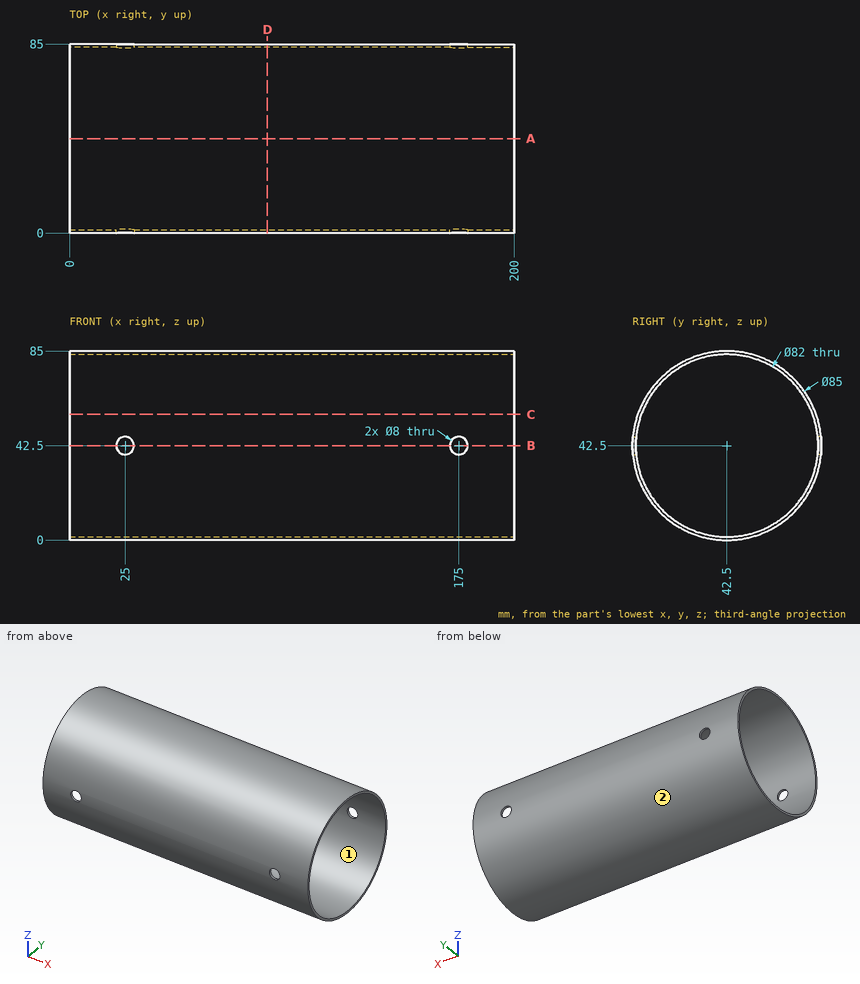
Could you check a few things on this drawing? It's one solid part, dimensions in mm from its lowest x, y, z. Coordinates: 2 decimals unless noted, no trailing zeros. Order: outer loops, then holes, each group sorted by start corner. A loop starts at its lowest first (then second) coordinate and runs counter-clockwise, first axis right, second up. Notation, with made-up numbers: M -34.5,45 L -26.5,45 A11 ccw -26.5,61 Z; hole C 72.5,42 d5. An arc over 180 degrees is marked long. Answer as a JSON object with one key per item and string values. Group by question number.
(1) Suppose I cut it at A-A, the plane y = 42.5. Please give me the cut outline in (x, z), then the cut area to 3 significant figures.
(2) Suppose I cut it at B-B, the plane z = 42.5. Please give me the cut outline in (x, y).
(3) Suppose I cut it at C-C, the plane z = 56.5. Please give me the cut outline in (x, y), then the cut area to 3 significant figures.
(4) I need wall thicknesses on probe 1 along X at (y, z) = (84, 42); probe 2 along Y at (x, z) = (9.5, 25); probe 3 along Z at (x, y) = (154, 64). Which ranges of each line are inside material? Lowest first, please.
(5) For pin 1 (5 mm diameter, centred on x = 167, z = 63, fed in from +Y); pin 2 (5 mm diameter, centred on x = 175, z = 42.5, fed in from +Y); pin 3 (12 mm diameter, centred on x = 171.5, y = 74, fed in from +Z); pin 4 (12 mm diameter, centred on x = 20.5, y = 70.5, fed in from +Z), each with a flat end and sliding along its axis, tell me the tip position at first contact or that it passes through.
(6) If we mould it in two halves opening along Z, with no side actions, what happens to the marked faces 1 and 2? For each: released by +Z, released by -Z, zero draft, split by the parting line, or undercut.
(7) Suppose I cut it at D-D, the plane x = 89. Please give me the cut outline in (y, z).
Values found:
{
 "1": {"outline": "M 0,0 L 200,0 L 200,1.5 L 0,1.5 Z; M 0,83.5 L 200,83.5 L 200,85 L 0,85 Z", "area": "600 mm^2"},
 "2": {"outline": "M 0,0 L 21,0 L 21,1.5 L 0,1.5 Z; M 0,83.5 L 21,83.5 L 21,85 L 0,85 Z; M 29,0 L 171,0 L 171,1.5 L 29,1.5 Z; M 29,83.5 L 171,83.5 L 171,85 L 29,85 Z; M 179,0 L 200,0 L 200,1.5 L 179,1.5 Z; M 179,83.5 L 200,83.5 L 200,85 L 179,85 Z"},
 "3": {"outline": "M 0,2.37 L 200,2.37 L 200,3.96 L 0,3.96 Z; M 0,81.04 L 200,81.04 L 200,82.63 L 0,82.63 Z", "area": "637 mm^2"},
 "4": {"probe 1": "x = 0 to 21.03, 28.97 to 171.03, 178.97 to 200", "probe 2": "y = 3.77 to 5.42, 79.58 to 81.23", "probe 3": "z = 5.84 to 7.59, 77.41 to 79.16"},
 "5": {"pin 1": "stops at y = 81", "pin 2": "passes through", "pin 3": "stops at z = 76.5", "pin 4": "stops at z = 78.86"},
 "6": {"face 1": "undercut", "face 2": "split by the parting line"},
 "7": {"outline": "C 42.5,42.5 d85; hole C 42.5,42.5 d82"}
}
